Input: dimensioned drawing with shaded views. Units: mm. Origin: part minimum x, y, z. A direction names the side the tool comes from. Round coordinates to 2 decimals unless told otherwise and drop trailing zeros. Loops run counter-clockwise (first coordinate to the right, second up) from the corner with the lowest first, then second, coordinate; pieces in that order, holes last. Notation, with made-up numbers: M -20.75,54.5 L 3.25,54.5 A17 cw 3.25,65.5 Z; hole C -39,11.5 d5. An arc over 180 degrees is marked long. Put each result on its own line as item: value. Start each with the question number.
1) Draft query along Y for the marked faces 1, 2 and 3. Return one class per face: +Y half, -Y half, draft (parallel to the pull), parting line (faces both ways), or undercut.
2) Section B-B on x = 8. State how many separate pieces and enclosed holes the cut face has.
3) Line query: probe 1 along Y at (x, z) = (8, 0.45); probe 2 along Y at (x, z) = (8, 2.25); probe 3 along Z at (x, y) = (14.5, 4.5). Output: solid intervals per line, ascending.
4) Section C-C on x = 2. Output: boundary loops of the cut face in (y, z).
5) Section A-A on y = 2.25. Output: boundary loops of the cut face in (x, z), plus the area to 3 significant figures.
6) Reachability of the marked faces 4 and 5 from +Z, -Z, +X, -X, +Y, -Y: full face, straight path, thin tool, end or side. Return the list, or none.
7) Pin query (flat end, axial travel): pin 1 (5 mm diameter, centred on y = 13, z = 7.5, fed in from -X); pin 2 (3 mm diameter, centred on x = 3.76, y = 12.24, fed in from +Z); pin 3 (2 mm diameter, centred on x = 6, z = 5, fed in from +Y); pin 4 (4 mm diameter, centred on y = 9.5, z = 16.5, fed in from -X). Return the tip coordinate at first contact, or that it passes through.
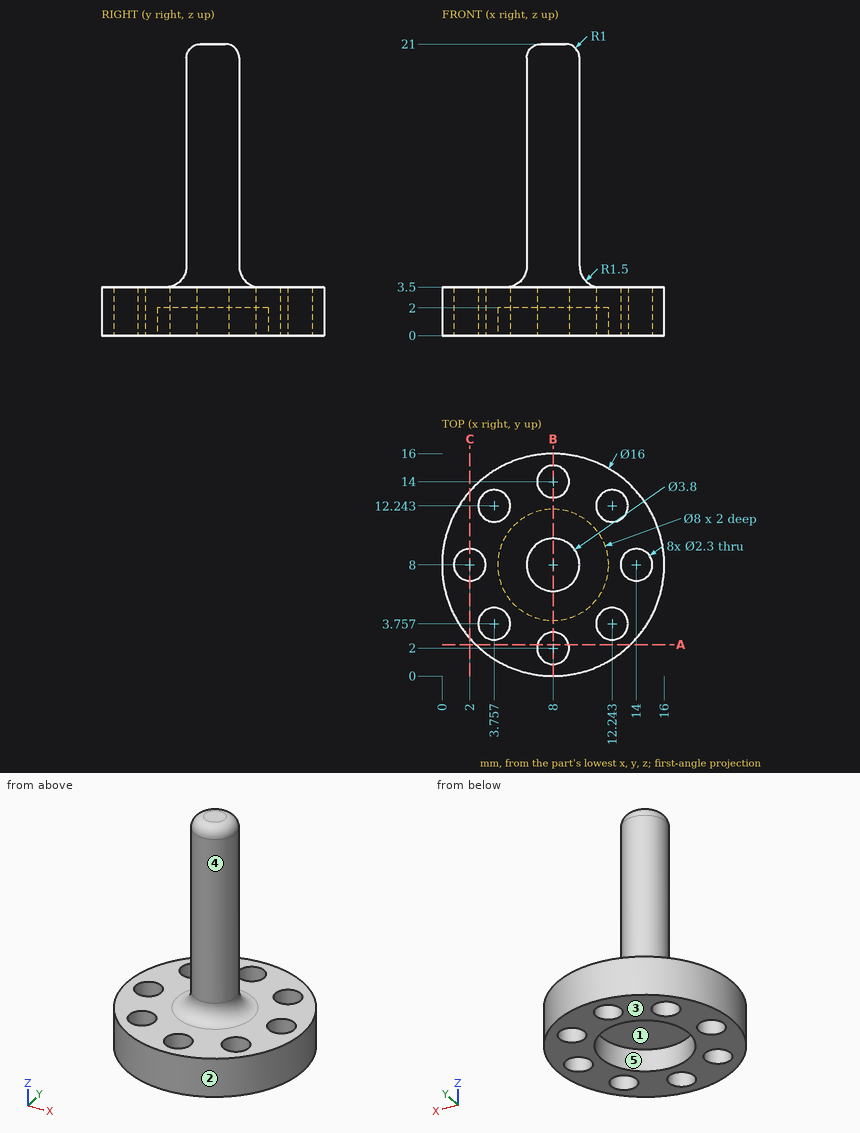
Geometry results:
1. face 1: undercut
1. face 2: parting line
1. face 3: draft
2. separate pieces: 3
2. enclosed holes: 0
3. probe 1: y = 0 to 0.85, 3.15 to 4, 12 to 12.85, 15.15 to 16
3. probe 2: y = 0 to 0.85, 3.15 to 12.85, 15.15 to 16
3. probe 3: z = 0 to 3.5
4. outline: M 2.71,0 L 6.85,0 L 6.85,3.5 L 2.71,3.5 Z; M 9.15,0 L 13.29,0 L 13.29,3.5 L 9.15,3.5 Z
5. outline: M 2.44,0 L 6.88,0 L 6.88,3.5 L 2.44,3.5 Z; M 9.12,0 L 13.56,0 L 13.56,3.5 L 9.12,3.5 Z
5. area: 31.1 mm²
6. face 4: +Z
6. face 5: -Z
7. pin 1: passes through
7. pin 2: stops at z = 3.5
7. pin 3: stops at y = 9.63
7. pin 4: stops at x = 6.1
